Can you work these out from the model? Positions are in its coordinate system, mm. Round coordinates to 2 decimals unless told otherwise and drop trailing zeros. Loops run counter-clockwise (first coordinate to the right, second up) from the corner with the lowest first, then second, coordinate; pieces in that order, holes last. Notation, with made-up numbers: M 27,44 L 86,44 A19 ccw 86,48 Z; hole C 70,67.25 d11. An arc over 180 degrees is marked long. Return JSON: item names as keys, results as strings.
```python
from build123d import *

# Parameters (mm, degrees)
SKETCH_1_R          = 35
EXTRUDE_1_DEPTH     = 7.5
FILLET_1_R          = 5
FILLET_2_R          = 5
SKETCH_2_R          = 15
CUT_EXTRUDE_1_DEPTH = 15
CHAMFER_1_SIZE      = 2
CHAMFER_2_SIZE      = 2
SCALE_1_SCALE       = 0.6


with BuildPart() as part:
    # 草图1 → 凸台-拉伸1 (new, symmetric)
    with BuildSketch(Plane.XY):
        Circle(SKETCH_1_R)
    extrude(amount=EXTRUDE_1_DEPTH, both=True)

    # 圆角1
    fillet_1_edges = [part.edges().sort_by_distance(p)[0] for p in [
        (-35, 0, 7.5),
    ]]
    fillet(fillet_1_edges, radius=FILLET_1_R)

    # 圆角2
    fillet_2_edges = [part.edges().sort_by_distance(p)[0] for p in [
        (-35, 0, -7.5),
    ]]
    fillet(fillet_2_edges, radius=FILLET_2_R)

    # 草图2 → 切除-拉伸1 (cut)
    with BuildSketch(Plane.XY.offset(7.5)):
        Circle(SKETCH_2_R)
    extrude(amount=-CUT_EXTRUDE_1_DEPTH, mode=Mode.SUBTRACT)

    # 倒角1
    chamfer_1_edges = [part.edges().sort_by_distance(p)[0] for p in [
        (-15, 0, 7.5),
    ]]
    chamfer(chamfer_1_edges, length=CHAMFER_1_SIZE)

    # 倒角2
    chamfer_2_edges = [part.edges().sort_by_distance(p)[0] for p in [
        (-15, 0, -7.5),
    ]]
    chamfer(chamfer_2_edges, length=CHAMFER_2_SIZE)


with BuildPart() as part_1:
    # 缩放比例1: scaled about (0, 0, 0)
    add(part.part.scale(SCALE_1_SCALE))


solid = part_1.part
```
Q1. If I drill on line 1 along Y through (x, z) = (0, 1); line 2 along Y through (x, z) = (5, 2); line 3 along X through (y, z) = (-1.5, 0.25), over which ranges is the centre line in solid material (lowest first)?
Results:
{"line 1": "y = -21 to -9, 9 to 21", "line 2": "y = -20.35 to -7.48, 7.48 to 20.35", "line 3": "x = -20.95 to -8.87, 8.87 to 20.95"}
Q2. Thinking about a two-plate mould opening in Y: for faces 1 (the cylindrical face through (20.03, 6.31, 0.02)), 2 (the cylindrical face through (-1.172, 8.923, 0.046)), 3 (the flat face through (8, -8, 4.5)), which applies, pulls with the +Y half, pulls with the -Y half, needs draft (parallel to the pull), parting line crosses it, or undercut?
Results:
{"face 1": "parting line crosses it", "face 2": "undercut", "face 3": "needs draft"}
Q3. Suppose I cut it at A-A, the plane x = 0. Please give me the cut outline in (y, z).
Results:
{"outline": "M -21,-1.5 A3 ccw -18,-4.5 L -10.2,-4.5 L -9,-3.3 L -9,3.3 L -10.2,4.5 L -18,4.5 A3 ccw -21,1.5 Z; M 9,-3.3 L 10.2,-4.5 L 18,-4.5 A3 ccw 21,-1.5 L 21,1.5 A3 ccw 18,4.5 L 10.2,4.5 L 9,3.3 Z"}
Q4. I'm going to push flat-ended pins straight in: pin 1 Ø3 at (x, z) = (-2, 0.5) entering from -Y; pin 2 Ø4 at (y, z) = (-6.5, 3) entering from +X; pin 3 Ø5 at (y, z) = (3.5, 0) entering from +X; pin 4 Ø16 at (x, y) = (0, 0) entering from -Z. Where does each tip first touch, or does it pass through?
Results:
{"pin 1": "stops at y = -20.99", "pin 2": "stops at x = 20.41", "pin 3": "stops at x = 20.98", "pin 4": "passes through"}
